Work out the finished part from the listing and answer in its coordinate system (mm). A direction names the side the tool comes from. Coordinates: 2 decimals unless noted, no trailing zeros. Loops run counter-clockwise (first coordinate to the right, second up) from the corner with the lowest first, then second, coordinate; pieces in that order, holes last. Notation, with made-up numbers: M 28.25,38.25 L 78.25,38.25 A16 cw 78.25,68.25 Z; hole C 2.25,68 d10. An arc over 180 degrees is marked long. Write each question's results on one line, items separated by ' | '.
Autodesk Inventor part; units mm, degrees
ref_plane "YZ Plane" through (0, 0, 0) normal (1, 0, 0) x (0, 1, 0)
ref_plane "XZ Plane" through (0, 0, 0) normal (0, 1, 0) x (-1, 0, 0)
ref_plane "XY Plane" through (0, 0, 0) normal (0, 0, 1) x (1, 0, 0)
sketch "Sketch1" plane through (0, 0, 0) normal (0, 0, 1) x (1, 0, 0)
  line L0 (21.8129, 13.019) -> (22.1812, -12.381)
  line L1 (22.1812, -12.381) -> (0.3684, -25.4)
  line L2 (0.3684, -25.4) -> (-21.8129, -13.019)
  line L3 (-21.8129, -13.019) -> (-22.1812, 12.381)
  line L4 (-22.1812, 12.381) -> (-0.3684, 25.4)
  line L5 (-0.3684, 25.4) -> (21.8129, 13.019)
  point P0 (0, 0)
  point P1 (0, 0)
  dimension "d0" = 25.4
  dimension "d1" = 120
extrude "Extrusion1" add sketch "Sketch1" along normal blind 35.56
sketch "Sketch2" plane through (0, 0, 35.56) normal (0, 0, 1) x (1, 0, 0)
  circle A0 centre (0, 0) radius 19.05
  dimension "d4" = 38.1
extrude "Extrusion2" cut sketch "Sketch2" against normal blind 30.48
sketch "Sketch3" plane through (0, 0, 0) normal (0, 0, -1) x (-1, 0, 0)
  circle A0 centre (0, 0) radius 10.922
  dimension "d7" = 21.844
extrude "Extrusion3" add sketch "Sketch3" along normal blind 19.05
thread "Thread1"
thread "Thread2"
properties part number "adapter"
1) Find section D-D, the plane z = -8. Give the vertices of the cut face in (x, y).
Check result:
outline: C 0,0 d21.84
2) Given pin 1 Ø10 at (x, z) = (-11.5, 19) entering from +Y; pin 2 Ø1 at (y, z) = (8, 18.5) entering from -X; pin 3 Ø8 at (x, z) = (-17.5, -13) entering from -Y; pin 4 Ø1 at (x, z) = (7.5, 1) entering from +Y, each flat-ended and moving along its own axis, determine where each tip first touches the part or whether it passes through.
Check result:
pin 1: y = 21.74 | pin 2: x = -22.12 | pin 3: through | pin 4: y = 21.29
3) Find section A-A, the plane z = 7. Give the vertices of the cut face in (x, y).
Check result:
outline: M -22.18,12.38 L -21.81,-13.02 L 0.37,-25.4 L 22.18,-12.38 L 21.81,13.02 L -0.37,25.4 Z; hole C 0,0 d38.1
4) Find section C-C, the plane y = 17. Give the vertices of the cut face in (x, z).
Check result:
outline: M -14.44,0 L 14.68,0 L 14.68,35.56 L 8.6,35.56 L 8.6,5.08 L -8.6,5.08 L -8.6,35.56 L -14.44,35.56 Z
5) Which of the six approach directions +Z, -Z, +X, -X, +Y, -Y give full straight-line access (tool end or side, diameter ignored) to faces 4 (the face through (-10, -5, 0)), 5 (the face through (0, 0, 5.08)), 6 (the face through (-11.43, 18.8, 17.53))?
Check result:
face 4: -Z | face 5: +Z | face 6: +Z, -Z, -X, +Y
6) Straight lines are drawn through the part: probe 1 along Z at (x, y) = (-5.5, 4.5); probe 2 along Z at (x, y) = (-15, 7); probe 3 along Y at (x, z) = (-14, 28.5). For each, find the intervals that lie inside material, in ascending order. Write a range as [from, to].
Check result:
probe 1: [-19.05, 5.08] | probe 2: [0, 5.08] | probe 3: [-17.38, -12.92], [12.92, 17.26]
7) For a pull along Y with two mould halves and no side action, classify faces 1 (the face through (-10.567, -19.296, 17.531)), 2 (the face through (-15.12, -11.59, 20.53)), 3 (the face through (0, 0, -19.05)) as released by +Y, released by -Y, zero draft, split by the parting line, or undercut.
Check result:
face 1: released by -Y | face 2: undercut | face 3: zero draft
8) Find section B-B, the plane x = 9.5. Give the vertices of the cut face in (y, z).
Check result:
outline: M -19.95,0 L -5.39,0 L -5.39,-19.05 L 5.39,-19.05 L 5.39,0 L 19.89,0 L 19.89,35.56 L 16.51,35.56 L 16.51,5.08 L -16.51,5.08 L -16.51,35.56 L -19.95,35.56 Z
